```python
from build123d import *

# Parameters (mm, degrees)
F0_W           = 30
F0_H           = 100
F1_DEPTH       = 5
F0_W_2         = 20
F2_DEPTH       = 10
F2_DEPTH_BACK  = 5
F4_D           = 5
F4_DEPTH       = 30
F4_CBORE_D     = 10
F4_CBORE_DEPTH = 5
F4_TIP         = 1.5021515476


with BuildPart() as f1:
    # F0 (on Top) → F1 (new body)
    with BuildSketch(Plane.XY):
        with Locations((-57.9909870028, 17.9872823166)):
            Rectangle(F0_W, F0_H)
        with Locations((-27.9909870028, 17.9872823166)):
            Rectangle(F0_W, F0_H)
    extrude(amount=F1_DEPTH)

    # F0 (on Top) → F2 (join, two sides)
    with BuildSketch(Plane.XY) as f2_sk:
        with Locations((-82.9909870028, 17.9872823166)):
            Rectangle(F0_W_2, F0_H)
        with Locations((-2.9909870028, 17.9872823166)):
            Rectangle(F0_W_2, F0_H)
    extrude(amount=-F2_DEPTH)
    extrude(f2_sk.sketch, amount=F2_DEPTH_BACK)

    # F4
    with Locations(Plane.XY.offset(5)):
        with Locations((-82.9909870028, -12.0127176834), (-82.9909870028, 47.9872823166), (-2.9909870028, 47.9872823166), (-2.9909870028, -12.0127176834)):
            CounterBoreHole(F4_D / 2, F4_CBORE_D / 2, F4_CBORE_DEPTH, depth=F4_DEPTH)
            with Locations((0, 0, -(F4_DEPTH + F4_TIP / 2))):  # 118° drill point
                Cone(0, F4_D / 2, F4_TIP, mode=Mode.SUBTRACT)


solid = f1.part
```
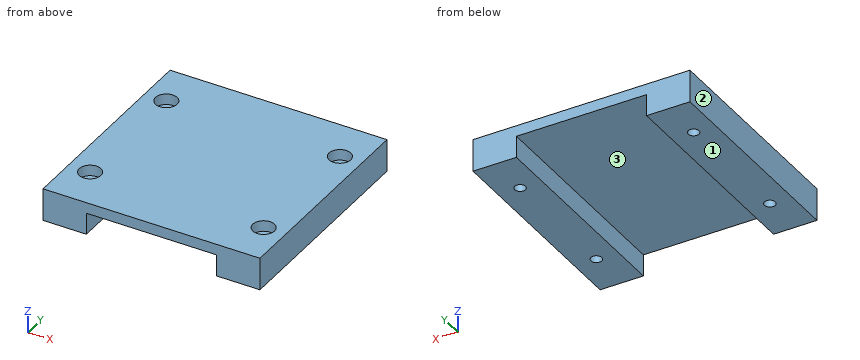
The model under review builds one solid part; all positions refer to its coordinate system, in mm. Face numbers are marked on the shaded views. Give positions to 0.01 mm unless a question says otherwise; leave off trailing zeros. Write each loop counter-clockwise with the first axis right and the second up, starting at its lowest first coordinate (ties: lowest second). Pieces come first, ordered by that corner, then holes. Notation, with made-up numbers: M -33.75,74.25 L 22.25,74.25 A3 ccw 22.25,78.25 Z; hole C -6,50.5 d7. An arc over 180 degrees is marked long. Answer in a Markdown table with one row per item.
Item 1: Add section D-D on z = 1.5. Give the boundary of the cut face in (x, y).
Check sheet entries:
| item | result |
|---|---|
| outline | M -92.99,-32.01 L 7.01,-32.01 L 7.01,67.99 L -92.99,67.99 Z; hole C -82.99,-12.01 d10; hole C -82.99,47.99 d10; hole C -2.99,-12.01 d10; hole C -2.99,47.99 d10 |
Item 2: Add section B-B on x = -2.5. Give the boundary of the cut face in (y, z).
Check sheet entries:
| item | result |
|---|---|
| outline | M -32.01,-10 L -14.46,-10 L -14.46,0 L -16.99,0 L -16.99,5 L -32.01,5 Z; M -9.56,-10 L 45.54,-10 L 45.54,0 L 43.01,0 L 43.01,5 L -7.04,5 L -7.04,0 L -9.56,0 Z; M 50.44,-10 L 67.99,-10 L 67.99,5 L 52.96,5 L 52.96,0 L 50.44,0 Z |
Item 3: For line 1 along X through (y, z) = (44.5, -1); line 2 along Y through (x, z) = (-1, 0.75); line 3 along X through (y, z) = (51.5, 4), list the stretches that pass through material, from the lowest coordinate up.
Check sheet entries:
| item | result |
|---|---|
| line 1 | -92.99 to -72.99, -12.99 to 7.01 |
| line 2 | -32.01 to -16.6, -7.43 to 43.4, 52.57 to 67.99 |
| line 3 | -92.99 to -86.55, -79.43 to -6.55, 0.57 to 7.01 |
Item 4: Add section A-A on z = -5.25. Give the boundary of the cut face in (x, y).
Check sheet entries:
| item | result |
|---|---|
| outline | M -92.99,-32.01 L -72.99,-32.01 L -72.99,67.99 L -92.99,67.99 Z; M -12.99,-32.01 L 7.01,-32.01 L 7.01,67.99 L -12.99,67.99 Z; hole C -82.99,-12.01 d5; hole C -82.99,47.99 d5; hole C -2.99,-12.01 d5; hole C -2.99,47.99 d5 |
Item 5: Draft analysis for pull direction X (two halves, no side actions). For the marked faces 1, 2 and 3, state which applies: +X half, -X half, draft (parallel to the pull), parting line (faces both ways), or undercut.
Check sheet entries:
| item | result |
|---|---|
| face 1 | draft |
| face 2 | -X half |
| face 3 | undercut |
Item 6: For P1, Ø5, axis at x = -3, y = 46, coming from the +Z side; P2, Ø6, axis at x = -67, y = 35, coming from the -Z side, all flat-tipped, find the tip position at first contact; note any pin that passes through.
Check sheet entries:
| item | result |
|---|---|
| P1 | z = 0 |
| P2 | z = 0 |
Item 7: Add section C-C on y = 40. Give the boundary of the cut face in (x, z).
Check sheet entries:
| item | result |
|---|---|
| outline | M -92.99,-10 L -72.99,-10 L -72.99,0 L -12.99,0 L -12.99,-10 L 7.01,-10 L 7.01,5 L -92.99,5 Z |
